Verification items for the finished model (mm, model axes). A direction names the side the tool comes from. Coordinates: 2 decimals unless noted, no trailing zeros. Order: outer loops, then holes, each group sorted by start corner. A loop starts at its lowest first (then second) coordinate and runs counter-clockwise, first axis right, second up.
Q1. Depth check by flat-ended pin: P1, Ø1.1, axis at y = 82, z = 52.5, coming from the +X side; P2, Ø9.5, axis at x = 15, z = 44, coming from the -Y side; P3, Ø4, axis at y = -9, z = 26, coming from the -X side. Enter the tip coordinate at first touch or a pass-through.
Q2. Cross-section at A-A, the plane z = 49. Record the boundary of the cut face in (x, y), and give its area (3 significant figures).
Q3. Thickness scan on line 1 (Y direction, x = 47.5, z = 49.5); line 2 (Z direction, x = 40.5, y = 56); line 3 (Y direction, x = -12, z = 85). Record the ranges inside material, lowest first.
Q4. Set-up check for faces 1 (the flat face through (-45, 78, 56)), 2 (the cylindrical face through (-13.401, 63.165, 52.507)), 3 (the cylindrical face through (84.594, -99.719, 46.084)), 4 (the cylindrical face through (-75.837, 92.138, 52.507)), 5 (the flat face through (-87, -1, 46)): record each of +Z, -Z, +X, -X, +Y, -Y from which the full face is reachable in a straight line by a thin tool's end or side.
Q5. Cross-section at C-C, the plane z = 28. Record the boundary of the cut face in (x, y), and give its area (3 significant figures).
from build123d import *

# Parameters (mm, degrees)
F0_W     = 180
F0_H     = 210
F1_DEPTH = 40
F2_W     = 186
F2_H     = 10
F3_DEPTH = 100
F4_W     = 174
F4_H     = 204
F5_DEPTH = 12
F6_W     = 65.3649838641
F6_H     = 31.9020412862
F7_DEPTH = 4
F8_DEPTH = 4
F9_R     = 8
F10_R    = 3
F11_R    = 2.99999
F12_R    = 5
F13_R    = 3


# Not quite as in the source:
# - a fillet or chamfer is up to 0.001 mm smaller than in the source, because OpenCascade refuses the exact size


with BuildPart() as f1:
    # F0 (on Top) → F1 (new body)
    with BuildSketch(Plane.XY):
        Rectangle(F0_W, F0_H)
    extrude(amount=F1_DEPTH)

    # F2 (on Top) → F3 (join)
    with BuildSketch(Plane.XY):
        with Locations((0, 110)):
            Rectangle(F2_W, F2_H)
    extrude(amount=F3_DEPTH)

    # F4 (on face) → F5 (join)
    with BuildSketch(Plane.XY.offset(40)):
        Rectangle(F4_W, F4_H)
    extrude(amount=F5_DEPTH)

    # F6 (on face) → F7 (join)
    with BuildSketch(Plane.XY.offset(52)):
        with Locations((-44.6581854485, 77.6125434786)):
            Rectangle(F6_W, F6_H)
    extrude(amount=F7_DEPTH)

    # F6 (on face) → F8 (join)
    with BuildSketch(Plane.XY.offset(52)):
        with Locations((-44.6581854485, 77.6125434786)):
            Rectangle(F6_W, F6_H)
        with Locations((44.6581854485, 77.6125434786)):
            Rectangle(F6_W, F6_H)
    extrude(amount=F8_DEPTH)

    # F9
    f9_edges = [f1.edges().sort_by_distance(p)[0] for p in [
        (-87, -102, 46),
        (87, -102, 46),
        (87, 102, 46),
        (-87, 102, 46),
    ]]
    fillet(f9_edges, radius=F9_R)

    # F10
    f10_edges = [f1.edges().sort_by_distance(p)[0] for p in [
        (-93, 110, 100),
        (-93, 105, 50),
        (0, 105, 100),
        (93, 105, 50),
        (93, 110, 100),
        (0, 115, 100),
        (-93, 115, 50),
        (93, 115, 50),
    ]]
    fillet(f10_edges, radius=F10_R)

    # F11 (radius 3 in the source; OpenCascade refuses exactly that, so slightly less here)
    f11_edges = [f1.edges().sort_by_distance(p)[0] for p in [
        (-90, 0, 40),
        (0, -105, 40),
        (-90, -105, 20),
        (90, -105, 20),
        (90, 0, 40),
    ]]
    fillet(f11_edges, radius=F11_R)

    # F12
    f12_edges = [f1.edges().sort_by_distance(p)[0] for p in [
        (-77.340677, 61.661523, 54),
        (-11.975694, 61.661523, 54),
        (-11.975694, 93.563564, 54),
        (-77.340677, 93.563564, 54),
        (11.975694, 93.563564, 54),
        (11.975694, 61.661523, 54),
        (77.340677, 61.661523, 54),
        (77.340677, 93.563564, 54),
    ]]
    fillet(f12_edges, radius=F12_R)

    # F13
    f13_edges = [f1.edges().sort_by_distance(p)[0] for p in [
        (77.340677, 77.612543, 56),
        (75.876211, 63.125989, 56),
        (75.876211, 92.099098, 56),
        (44.658185, 61.661523, 56),
        (44.658185, 93.563564, 56),
        (13.44016, 63.125989, 56),
        (13.44016, 92.099098, 56),
        (11.975694, 77.612543, 56),
        (-44.658185, 93.563564, 56),
        (-13.44016, 92.099098, 56),
        (-75.876211, 92.099098, 56),
        (-11.975694, 77.612543, 56),
        (-77.340677, 77.612543, 56),
        (-13.44016, 63.125989, 56),
        (-75.876211, 63.125989, 56),
        (-44.658185, 61.661523, 56),
    ]]
    fillet(f13_edges, radius=F13_R)


solid = f1.part
Check values:
1. P1: stops at x = 87
1. P2: stops at y = -103.98
1. P3: stops at x = -90
2. outline: (-93, 108) arc R3 ccw to (-90, 105) - (90, 105) arc R3 ccw to (93, 108) - (93, 112) arc R3 ccw to (90, 115) - (-90, 115) arc R3 ccw to (-93, 112) - close; (-87, -94) arc R8 ccw to (-79, -102) - (79, -102) arc R8 ccw to (87, -94) - (87, 94) arc R8 ccw to (79, 102) - (-79, 102) arc R8 ccw to (-87, 94) - close
2. area: 37,300 mm2
3. line 1: y = -102 to 102, 105 to 115
3. line 2: z = 0 to 52
3. line 3: y = 105 to 115
4. face 1: +Z, +X, -X, -Y
4. face 2: +Z, -Y
4. face 3: +Z, +X, -Y
4. face 4: +Z, -X
4. face 5: +Z, -X, -Y
5. outline: (-93, 108) arc R3 ccw to (-90, 105) - (-90, -102) arc R3 ccw to (-87, -105) - (87, -105) arc R3 ccw to (90, -102) - (90, 105) arc R3 ccw to (93, 108) - (93, 112) arc R3 ccw to (90, 115) - (-90, 115) arc R3 ccw to (-93, 112) - close
5. area: 39,600 mm2
